Here's how the part is built. I have some questions about the finished solid (model axes, mm). Face numbers are marked on the shaded views. Round coordinates to 2 decimals unless told otherwise and drop trailing zeros. Order: outer loops, then holes, each group sorted by start corner. A loop starts at its lowest first (then second) coordinate and runs counter-clockwise, first axis right, second up.
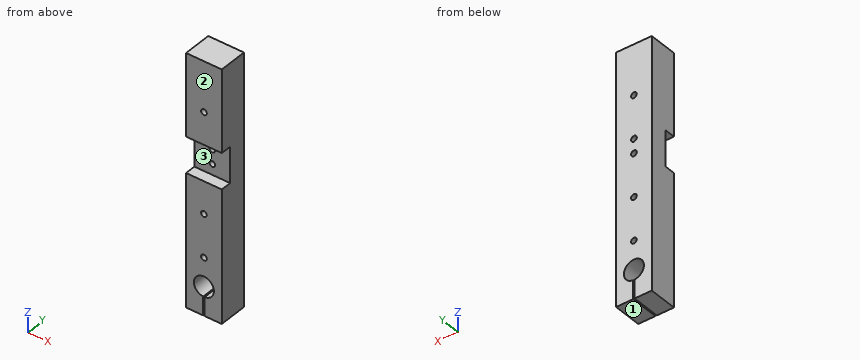
```python
from build123d import *

# Parameters (mm, degrees)
EXTRUDE_1_DEPTH     = 40
SKETCH_2_R          = 4
CUT_EXTRUDE_1_DEPTH = 50
SKETCH_3_W          = 50
SKETCH_3_H          = 50
CUT_EXTRUDE_2_DEPTH = 15


with BuildPart() as part:
    # Эскиз1 → Бобышка-Вытянуть1 (new body)
    with BuildSketch(Plane(origin=(0, 0, 0), x_dir=(1, 0, 0), z_dir=(0, 1, 0))):
        with BuildLine():
            Line((0, 0), (50, 0))
            Line((50, 0), (50, 350))
            Line((50, 350), (26, 350))
            Line((26, 350), (26, 323.964240044))
            ThreePointArc((26, 323.964240044), (25, 296), (24, 323.964240044))
            Line((24, 323.964240044), (24, 350))
            Line((24, 350), (0, 350))
            Line((0, 350), (0, 0))
        make_face()
    extrude(amount=EXTRUDE_1_DEPTH)

    # Эскиз2 → Вырез-Вытянуть1 (cut)
    with BuildSketch(Plane(origin=(0, 40, 0), x_dir=(1, 0, 0), z_dir=(0, 1, 0))):
        with Locations(Location((25, 130, 0), (0, 0, 270))):
            Circle(SKETCH_2_R)
        with Locations(Location((25, 150, 0), (0, 0, 270))):
            Circle(SKETCH_2_R)
        with Locations(Location((25, 270, 0), (0, 0, 270))):
            Circle(SKETCH_2_R)
        with Locations(Location((25, 210, 0), (0, 0, 270))):
            Circle(SKETCH_2_R)
        with Locations(Location((25, 70, 0), (0, 0, 270))):
            Circle(SKETCH_2_R)
    extrude(amount=-CUT_EXTRUDE_1_DEPTH, mode=Mode.SUBTRACT)

    # Эскиз3 → Вырез-Вытянуть2 (cut)
    with BuildSketch(Plane.XZ):
        with Locations((25, -140)):
            Rectangle(SKETCH_3_W, SKETCH_3_H)
    extrude(amount=-CUT_EXTRUDE_2_DEPTH, mode=Mode.SUBTRACT)


solid = part.part
```
1. If we mould it in two halves opening along Z, with no side actions, what happens to the marked faces 1, 2 and 3? For each: released by +Z, released by -Z, zero draft, split by the parting line, or undercut.
Evaluation:
face 1: released by -Z
face 2: zero draft
face 3: undercut
2. If we section it at C-C, the plane x = 45.5: Write out the boundary of the cut face in (y, z).
Evaluation:
outline: (0, -350) - (40, -350) - (40, 0) - (0, 0) - (0, -115) - (15, -115) - (15, -165) - (0, -165) - close
3. I need wall thicknesses on probe 1 along Z at (x, y) = (7, 6); probe 2 along X at (y, z) = (29, -150); probe 3 along X at (y, z) = (21, -310). Which ranges of each line are inside material? Lowest first, please.
Evaluation:
probe 1: z = -350 to -165, -115 to 0
probe 2: x = 0 to 21, 29 to 50
probe 3: x = 0 to 11, 39 to 50
4. If we section it at D-D, the plane y = 28: Write out the boundary of the cut face in (x, z), and give its area (3 significant figures).
Evaluation:
outline: (0, -350) - (24, -350) - (24, -323.96) arc R14 cw (long way) to (26, -323.96) - (26, -350) - (50, -350) - (50, 0) - (0, 0) - close; hole circle Ø8 at (25, -270); hole circle Ø8 at (25, -210); hole circle Ø8 at (25, -150); hole circle Ø8 at (25, -130); hole circle Ø8 at (25, -70)
area: 16,600 mm2
5. I'm going to push flat-ended pins straight in: P1, Ø13, axis at x = 25, z = -210, coming from the -Y side; P2, Ø25, axis at x = 28, z = -130, coming from the -Y side. Where does each tip first touch, or does it pass through?
Evaluation:
P1: stops at y = 0
P2: stops at y = 15
6. If we section it at A-A, the plane y = 3: Write out the boundary of the cut face in (x, z).
Evaluation:
outline: (0, -350) - (24, -350) - (24, -323.96) arc R14 cw (long way) to (26, -323.96) - (26, -350) - (50, -350) - (50, -165) - (0, -165) - close; (0, -115) - (50, -115) - (50, 0) - (0, 0) - close; hole circle Ø8 at (25, -270); hole circle Ø8 at (25, -210); hole circle Ø8 at (25, -70)
7. If we section it at B-B, the plane z = -70: Write out the boundary of the cut face in (x, y), and give its area (3 significant figures).
Evaluation:
outline: (0, 0) - (21, 0) - (21, 40) - (0, 40) - close; (29, 0) - (50, 0) - (50, 40) - (29, 40) - close
area: 1,680 mm2
